Autodesk Inventor part; units mm, degrees
ref_plane "YZ Plane" through (0, 0, 0) normal (1, 0, 0) x (0, 1, 0)
ref_plane "XZ Plane" through (0, 0, 0) normal (0, 1, 0) x (-1, 0, 0)
ref_plane "XY Plane" through (0, 0, 0) normal (0, 0, 1) x (1, 0, 0)
sketch "スケッチ1" plane through (0, 0, 0) normal (0, 0, 1) x (1, 0, 0)
  circle A0 centre (0, 0) radius 1.7
  circle A1 centre (48, 0) radius 1.7
  circle A2 centre (0, 0) radius 3
  circle A3 centre (48, 0) radius 3
  line L0 (0, 3) -> (48, 3)
  line L1 (0, -3) -> (48, -3)
  dimension "d0" = 3.4
  dimension "d1" = 3.4
  dimension "d2" = 6
  dimension "d3" = 6
  dimension "d4" = 48
extrude "押し出し1" add sketch "スケッチ1" along normal mid plane 4
offset faces "サイズ1" outward -0.05 faces at (49.6945, -0.1368, 0.6667)
offset faces "サイズ2" outward -0.05 faces at (1.6945, 0.1368, -0.6667)
scale "尺度1" factors (0.8836555, 0.8836555, 0.8836555) then translate (2.7923, 0.349, -0.2327) bodies 1
sketch "スケッチ2" plane through (2.7923, -2.3019, 1.5346) normal (0, 0, 1) x (1, 0, 0)
  circle A0 centre (0, 2.651) radius 1.5464
  circle A1 centre (0, 2.651) radius 1.65
  circle A2 centre (42.4155, 2.651) radius 1.5464
  circle A3 centre (42.4155, 2.651) radius 1.65
  point P0 (-2.7923, 2.3019)
  dimension "d12" = 3.3
extrude "押し出し2" cut sketch "スケッチ2" against normal up to next
sketch "スケッチ3" plane through (2.7923, -2.3019, 1.5346) normal (0, 0, 1) x (1, 0, 0)
  circle A0 centre (0, 2.651) radius 1.65
  circle A1 centre (42.4155, 2.651) radius 1.65
  arc A2 (0, 5.3019) -> (0, 0) centre (0, 2.651) ccw
  line L0 (0, 0) -> (42.4155, 0)
  arc A3 (42.4155, 0) -> (42.4155, 5.3019) centre (42.4155, 2.651) ccw
  line L1 (42.4155, 5.3019) -> (0, 5.3019)
  point P0 (-2.7923, 2.3019)
extrude "押し出し3" add sketch "スケッチ3" along normal blind 6
sketch "スケッチ4" plane through (2.7923, 3, -2) normal (0, 1, 0) x (1, 0, 0)
  line L0 (42.4155, -9.5346) -> (45.0664, -9.5346)
  line L1 (45.0664, -9.5346) -> (45.0664, -3.5346)
  line L2 (45.0664, 0) -> (45.0664, -9.5346)
  line L3 (45.0664, -3.5346) -> (17.4176, -3.5346)
  line L4 (-2.651, 0) -> (-2.651, -6)
  line L5 (-2.651, 0) -> (-2.651, -9.5346)
  line L6 (-2.651, -6) -> (12.349, -6)
  line L7 (12.349, -6) -> (15.0664, 0)
  line L8 (42.4155, 0) -> (0, 0)
  line L9 (15.0664, 0) -> (-2.651, 0)
  line L10 (17.4176, -3.5346) -> (14.7002, -9.5346)
  line L11 (14.7002, -9.5346) -> (45.0664, -9.5346)
  line L12 (42.4155, -9.5346) -> (0, -9.5346)
  line L13 (0, 0) -> (42.4155, 0)
  point P0 (-2.7923, -2)
  dimension "d17" = 6
  dimension "d18" = 6
  dimension "d20" = 3.6
  dimension "d21" = 30
  dimension "d22" = 15
extrude "押し出し4" cut sketch "スケッチ4" against normal through all
sketch "スケッチ5" plane through (2.7923, -2.3019, 7.5346) normal (0, 0, 1) x (1, 0, 0)
  circle A0 centre (0, 2.651) radius 1.65
  line L0 (0, 0) -> (14.7002, 0)
  arc A1 (0, 0) -> (2.6467, 2.5) centre (0, 2.651) ccw
  line L1 (2.6467, 2.5) -> (39.7688, 2.5)
  line L2 (0, 0) -> (42.4155, 0)
  line L3 (42.4155, 0) -> (15.0664, 0)
  arc A2 (39.7688, 2.5) -> (42.4155, 0) centre (42.4155, 2.651) ccw
  point P0 (-2.7923, 2.3019)
  dimension "d28" = 2.5
extrude "押し出し5" cut sketch "スケッチ5" against normal up to next contours A1 L1 A2 L2 L0
fillet "フィレット1" radius 1 2 edges at (42.5611, 0.1981, -0.2327) (5.4389, 0.1981, 5.7673)
sketch "スケッチ6" plane through (2.7923, -2.3019, 7.5346) normal (0, 0, 1) x (1, 0, 0)
  circle A0 centre (-5, 2.651) radius 1.65
  circle A1 centre (-5, 2.651) radius 2.651
  arc A2 (0, 5.3019) -> (2.5158, 1.8152) centre (0, 2.651) ccw
  circle A3 centre (0, 2.651) radius 1.65
  line L0 (-5, 0) -> (0, 0)
  arc A4 (0, 5.3019) -> (2.5158, 1.8152) centre (0, 2.651) ccw
  line L1 (12.349, 5.3019) -> (0, 5.3019)
  line L2 (-5, 5.3019) -> (0, 5.3019)
  arc A5 (0, 0) -> (0, 5.3019) centre (0, 2.651) ccw
  point P0 (-2.7923, 2.3019)
  dimension "d32" = 5
extrude "押し出し6" add sketch "スケッチ6" against normal up to surface (3.5346 mm away) contours A1 A2 | L2 A2 A1 | A1 A2 L0 | A2 A5 A1 | A1 A2 | A3
fillet "フィレット2" radius 2 2 edges at (20.2099, 1.599, 1.5346) (15.1413, 1.599, 4)
sketch "スケッチ7" plane through (17.8587, 3, -2) normal (0, 1, 0) x (1, 0, 0)
  line L0 (-0.3662, -9.5346) -> (1.8191, -4.7095)
  line L1 (1.3095, -5.8346) -> (15.3095, -5.8346)
  line L2 (15.3095, -5.8346) -> (16.3512, -3.5346)
  line L3 (3.6409, -3.5346) -> (23.8842, -3.5346)
  line L4 (16.3512, -3.5346) -> (2.3512, -3.5346)
  line L5 (2.3512, -3.5346) -> (1.3095, -5.8346)
  line L6 (-0.3662, -9.5346) -> (1.8191, -4.7095)
  point P0 (-17.8587, -2)
  dimension "d36" = 2.3
  dimension "d37" = 14
extrude "押し出し7" add sketch "スケッチ7" against normal up to surface (2.8019 mm away)
fillet "フィレット3" radius 2 2 edges at (19.1682, 1.599, 3.8346) (34.2099, 1.599, 1.5346)
sketch "スケッチ8" plane through (17.8587, 3, -2) normal (0, 1, 0) x (1, 0, 0)
  line L0 (0, 0) -> (27.349, 0)
  line L1 (14.6587, 0) -> (13.3749, -2.8346)
  line L2 (13.3749, -2.8346) -> (-1.2838, -2.8346)
  line L3 (0, 0) -> (-2.1853, -4.8251) construction
  line L4 (-1.2838, -2.8346) -> (0, 0)
  line L5 (0, 0) -> (14.6587, 0)
  line L6 (2.5993, -5.8346) -> (15.3095, -5.8346)
  line L7 (15.3095, -5.8346) -> (15.8191, -4.7095)
  point P0 (-17.8587, -2)
  dimension "d41" = 3
  dimension "d42" = 3
extrude "押し出し8" cut sketch "スケッチ8" against normal through all
fillet "フィレット4" radius 1.5 5 edges at (16.5749, 1.599, 0.8346) (31.2336, 1.599, 0.8346) (32.5174, 1.599, -2) (17.4925, 1.599, 7.5346) (33.1682, 1.599, 3.8346)
sketch "スケッチ9" plane through (2.7923, -2.3019, 7.5346) normal (0, 0, 1) x (1, 0, 0)
  circle A0 centre (-5, 2.651) radius 1.65
  circle A1 centre (-5, 2.651) radius 3.5
  point P0 (-2.7923, 2.3019)
  dimension "d46" = 7
extrude "押し出し9" add sketch "スケッチ9" against normal up to surface (3.5346 mm away)
sketch "スケッチ10" plane through (35.4996, 3, 1.5346) normal (0, 0, 1) x (1, 0, 0)
  circle A0 centre (9.7081, -2.651) radius 1.65
  circle A1 centre (9.7081, -2.651) radius 3.5
  point P0 (-35.4996, -3)
  dimension "d49" = 7
extrude "押し出し10" add sketch "スケッチ10" against normal up to surface (3.5346 mm away)
fillet "フィレット5" radius 2 2 edges at (42.9225, 3, -0.2327) (41.711, 0.1981, -0.2327)
properties part number "HbFingerMainCouplerLink01"
The listing builds one solid part. Answer for the finished solid, in the listing's coordinates (mm). A direction names the side the tool comes from. Give positions to 0.01 mm unless a question says otherwise; leave off trailing zeros. Write each loop counter-clockwise with the first axis right and the second up, starting at its lowest first coordinate (ties: lowest second). Pieces come first, ordered by that corner, then holes.
Item 1: Flat-ended cylindrical pins translate along their axes: P1, Ø5, axis at x = 23, z = 0.5, coming from the -Y side; P2, Ø1.5, axis at x = 30.5, z = 1.5, coming from the +Y side; P3, Ø1.6, axis at x = 43.5, y = -0.5, coming from the +Z side; P4, Ø4, axis at y = -1, z = -1, coming from the +X side. Find the tip coordinate at first contact, or state that the pin passes through.
Item 2: Section A-A, the plane y = 1.25 is taken. Write down the section's boundary in (x, z), plus the area to 3 significant figures.
Item 3: Which of the six approach directions +Z, -Z, +X, -X, +Y, -Y give full straight-line access (tool end or side, diameter ignored) to faces 1 (the flat face through (23, 0.198, 3)), 2 (the flat face through (31.88, 1.62, -0.59)), 3 (the flat face through (1, -2.302, 6))?
Item 4: Find the intervals of material crossed by line 1 along Y through (x, z) = (25, 1); line 2 along Y through (x, z) = (45, -0.5); line 3 along Z through (x, y) = (5, 1.5), in increasing order.
Item 5: Determine the mould class of faces 4 (the cylindrical face through (-3.856, 0.422, 5.792)), 5 (the cylindrical face through (14.95, 1.58, 3.67)), 6 (the flat face through (24, 2, 0.835)), 7 (the cylindrical face through (4.325, -1.814, 5.792)) for opening direction X: released by +X, released by -X, zero draft, split by the parting line, or undercut.
Item 6: Section D-D, the plane x = 2 is taken. Write down the section's boundary in (y, z).
Item 7: Section B-B, the plane x = 12.5 is taken. Write down the section's boundary in (y, z), plus the area to 3 significant figures.
Item 8: Section C-C, the plane z = 6 is taken. Write down the section's boundary in (x, y).
Completed:
1. P1: stops at y = 0.2
1. P2: stops at y = 3
1. P3: stops at z = 1.53
1. P4: stops at x = 48.71
2. outline: (-5.59, 4) - (-3.59, 4) - (-3.59, 7.53) - (-5.59, 7.53) - close; (-0.83, 4) - (13.85, 4) arc R2 cw to (15.67, 2.83) - (16.18, 1.72) arc R1.5 ccw to (17.54, 0.83) - (30.27, 0.83) arc R1.5 cw to (31.63, -0.05) - (32.12, -1.12) arc R1.5 ccw to (33.48, -2) - (43.83, -2) - (43.83, 1.53) - (35.5, 1.53) arc R2 cw to (33.68, 2.71) - (33.57, 2.95) arc R1.5 ccw to (32.2, 3.83) - (20.46, 3.83) arc R2 cw to (18.64, 5.01) - (17.89, 6.65) arc R1.5 ccw to (16.53, 7.53) - (-0.83, 7.53) - close; (46.59, -2) - (48.59, -2) - (48.59, 1.53) - (46.59, 1.53) - close
2. area: 177 mm2
3. face 1: +Z, -Z, -Y
3. face 2: -Z, -X, +Y, -Y
3. face 3: +Z, -Z, +X, -Y
4. line 1: y = 0.2 to 3
4. line 2: y = -3.14 to -1.29, 1.99 to 3.84
4. line 3: z = 4 to 7.53
5. face 4: undercut
5. face 5: released by -X
5. face 6: zero draft
5. face 7: released by +X
6. outline: (-2.3, 4) - (3, 4) - (3, 7.53) - (-2.3, 7.53) - close
7. outline: (0.2, 4) - (3, 4) - (3, 7.53) - (0.2, 7.53) - close
7. area: 9.90 mm2
8. outline: (0.08, -2.3) - (2.79, -2.3) arc R2.65 ccw to (5.31, -0.49) arc R1 cw to (6.26, 0.2) - (18.19, 0.2) - (18.19, 3) - (0.08, 3) arc R3.5 ccw (long way) to start; hole circle Ø3.3 at (-2.21, 0.35)
